```python
from build123d import *
from OCP.BRepFilletAPI import BRepFilletAPI_MakeChamfer

# Parameters (mm, degrees)
ESTRUSIONE_ESTRUSIONE1_DEPTH = 20
SCHIZZO2_R                   = 4.5
TAGLIO_ESTRUSIONE1_DEPTH     = 40.449334595
SMUSSO1_SIZE                 = 1
SMUSSO1_SIZE2                = 0.577350269


with BuildPart() as part:
    # Schizzo1 → Estrusione-Estrusione1 (new body)
    with BuildSketch(Plane.XY):
        with BuildLine():
            Line((-8.5, 8.5), (-8.5, 0))
            Line((-8.5, 0), (-27.5, 0))
            Line((-27.5, 0), (-27.5, 20))
            Line((-27.5, 20), (27.5, 20))
            Line((27.5, 20), (27.5, 0))
            Line((27.5, 0), (8.5, 0))
            Line((8.5, 0), (8.5, 8.5))
            ThreePointArc((8.5, 8.5), (0, 17), (-8.5, 8.5))
        make_face()
    extrude(amount=ESTRUSIONE_ESTRUSIONE1_DEPTH)

    # Schizzo2 → Taglio-Estrusione1 (cut, through all)
    with BuildSketch(Plane.XZ):
        with Locations((-18, 10)):
            Circle(SCHIZZO2_R)
        with Locations((18, 10)):
            Circle(SCHIZZO2_R)
    extrude(amount=-TAGLIO_ESTRUSIONE1_DEPTH, mode=Mode.SUBTRACT)

    # Smusso1: one chamfer whose edges measure the first distance from different faces: ONE call of the kernel's chamfer builder (chamfer() names one face for all edges)
    smusso1_edges_1 = [part.edges().sort_by_distance(p)[0] for p in [
        (-27.5, 10, 20),
    ]]
    smusso1_side_1 = [part.faces().sort_by_distance(p)[0] for p in [
        (-27.5, 10, 10),
    ]]
    smusso1_edges_2 = [part.edges().sort_by_distance(p)[0] for p in [
        (0, 20, 0),
        (-27.5, 20, 10),
        (27.5, 20, 10),
        (0, 20, 20),
    ]]
    smusso1_side_2 = [part.faces().sort_by_distance(p)[0] for p in [
        (0, 20, 10),
    ]]
    smusso1_edges_3 = [part.edges().sort_by_distance(p)[0] for p in [
        (27.5, 10, 0),
        (-27.5, 10, 0),
    ]]
    smusso1_side_3 = [part.faces().sort_by_distance(p)[0] for p in [
        (-9.085234996, 4.25, 0),
    ]]
    smusso1_edges_4 = [part.edges().sort_by_distance(p)[0] for p in [
        (27.5, 10, 20),
    ]]
    smusso1_side_4 = [part.faces().sort_by_distance(p)[0] for p in [
        (27.5, 10, 10),
    ]]
    smusso1 = BRepFilletAPI_MakeChamfer(part.part.solid().wrapped)
    for e in smusso1_edges_1:
        smusso1.Add(SMUSSO1_SIZE, SMUSSO1_SIZE2, e.wrapped, smusso1_side_1[0].wrapped)  # the first distance lies on this face
    for e in smusso1_edges_2:
        smusso1.Add(SMUSSO1_SIZE, SMUSSO1_SIZE2, e.wrapped, smusso1_side_2[0].wrapped)  # the first distance lies on this face
    for e in smusso1_edges_3:
        smusso1.Add(SMUSSO1_SIZE, SMUSSO1_SIZE2, e.wrapped, smusso1_side_3[0].wrapped)  # the first distance lies on this face
    for e in smusso1_edges_4:
        smusso1.Add(SMUSSO1_SIZE, SMUSSO1_SIZE2, e.wrapped, smusso1_side_4[0].wrapped)  # the first distance lies on this face
    add(Compound.cast(smusso1.Shape()), mode=Mode.REPLACE)


solid = part.part
```
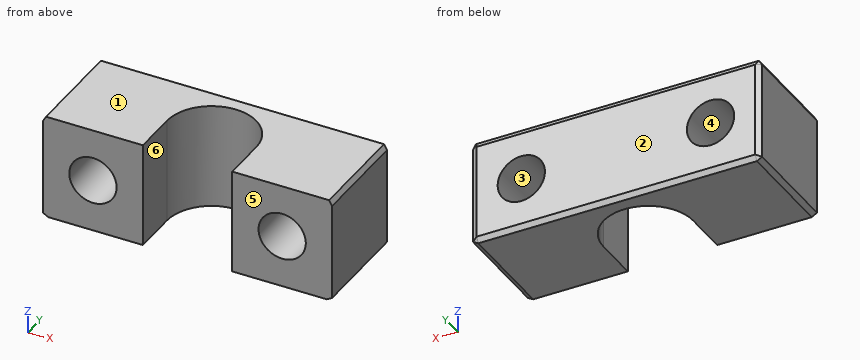
The model under review builds one solid part; all positions refer to its coordinate system, in mm. Face numbers are marked on the shaded views. A direction names the side the tool comes from. Round coordinates to 2 decimals unless told otherwise and drop trailing zeros. Loops run counter-clockwise (first coordinate to the right, second up) from the corner with the lowest first, then second, coordinate; pieces in that order, holes last. Notation, with made-up numbers: (13, 64) -> (33, 64) arc R14 cw to (33, 73) -> close; hole circle Ø2 at (45.25, 11.5). An arc over 180 degrees is marked (long way). Answer in a Markdown table with one row per item.
1) For pin 1 Ø7 at (x, z) = (18, 10) entering from +Y, flat-tipped, find the tip position at first contact; note if it passes through.
Taken from the geometry:
| item | result |
|---|---|
| pin 1 | passes through |
2) Tool access review of the marked faces 5 and 6: name each direction out of +Z, -Z, +X, -X, +Y, -Y from which nothing blocks a thin tool from reaching the whole face with its end or side.
Taken from the geometry:
| item | result |
|---|---|
| face 5 | +Z, -Z, +X, -X, -Y |
| face 6 | +Z, -Z, -Y |
3) Wall thickness on line 1 along X through (y, z) = (7.5, 2.75); line 2 along X through (y, z) = (1.75, 7.25); line 3 along Z through (x, y) = (18, 14.75): over which ranges is each line inside the solid? List them lowest first.
Taken from the geometry:
| item | result |
|---|---|
| line 1 | x = -27.5 to -8.5, 8.5 to 27.5 |
| line 2 | x = -27.5 to -21.56, -14.44 to -8.5, 8.5 to 14.44, 21.56 to 27.5 |
| line 3 | z = 0 to 5.5, 14.5 to 20 |
4) Consider section A-A, the plane y = 8. Write out the cut boundary in (x, z), plus the area to 3 significant figures.
Taken from the geometry:
| item | result |
|---|---|
| outline | (-27.5, 0.58) -> (-26.5, 0) -> (-8.5, 0) -> (-8.5, 20) -> (-26.92, 20) -> (-27.5, 19) -> close; (8.5, 0) -> (26.5, 0) -> (27.5, 0.58) -> (27.5, 19) -> (26.92, 20) -> (8.5, 20) -> close; hole circle Ø9 at (-18, 10); hole circle Ø9 at (18, 10) |
| area | 632 mm² |
5) Draft analysis for pull direction Z (two halves, no side actions). For the marked faces 1, 2, 3 and 4, state which applies: pulls with the +Z half, pulls with the -Z half, needs draft (parallel to the pull), parting line crosses it, or undercut.
Taken from the geometry:
| item | result |
|---|---|
| face 1 | pulls with the +Z half |
| face 2 | needs draft |
| face 3 | undercut |
| face 4 | undercut |
6) Consider section B-B, the plane x = -18. Write out the cut boundary in (y, z).
Taken from the geometry:
| item | result |
|---|---|
| outline | (0, 0) -> (19.42, 0) -> (20, 1) -> (20, 5.5) -> (0, 5.5) -> close; (0, 14.5) -> (20, 14.5) -> (20, 19) -> (19.42, 20) -> (0, 20) -> close |
7) Consider section D-D, the plane z = 4.75. Write out the cut boundary in (x, y), plus the area to 3 significant figures.
Taken from the geometry:
| item | result |
|---|---|
| outline | (-27.5, 0) -> (-8.5, 0) -> (-8.5, 8.5) arc R8.5 cw to (8.5, 8.5) -> (8.5, 0) -> (27.5, 0) -> (27.5, 19.42) -> (26.5, 20) -> (-26.5, 20) -> (-27.5, 19.42) -> close |
| area | 841 mm² |
8) Consider section C-C, the plane y = 18.75. Write out the cut boundary in (x, z).
Taken from the geometry:
| item | result |
|---|---|
| outline | (-27.5, 0.58) -> (-26.5, 0) -> (26.5, 0) -> (27.5, 0.58) -> (27.5, 19) -> (26.92, 20) -> (-26.92, 20) -> (-27.5, 19) -> close; hole circle Ø9 at (-18, 10); hole circle Ø9 at (18, 10) |
